Source: CAD feature listing. Evaluate the final solid. Frame: model axes, mm. Round coordinates to 2 decimals unless told otherwise and drop trailing zeros. Order: outer loops, then holes, each group sorted by start corner. A loop starts at its lowest first (then second) coordinate and runs counter-clockwise, first axis right, second up. Notation, with made-up numbers: M 17,74.5 L 56,74.5 A24 cw 56,84.5 Z; hole C 75,73.5 d2. An arc over 180 degrees is marked long. Use one line per item in the form item = value. Start each with the question number.
Q1. Section A-A (z = -131.5). Return the cut outline in (x, y).
Q2. Contact query for flat-ended pins moving along their axis: pin 1 (6 mm diameter, centred on x = 0, y = 0, fed in from +Z); pin 2 (6.5 mm diameter, centred on x = 0, z = 90, fed in from -Y). Output: stop coordinate, or through.
Q3. Material intervals for probe 1 along Y at (x, z) = (0, -138.5); probe 2 along X at (y, z) = (-1.25, 90); probe 3 along Z at (x, y) = (-0.5, -5), sorted ascending.
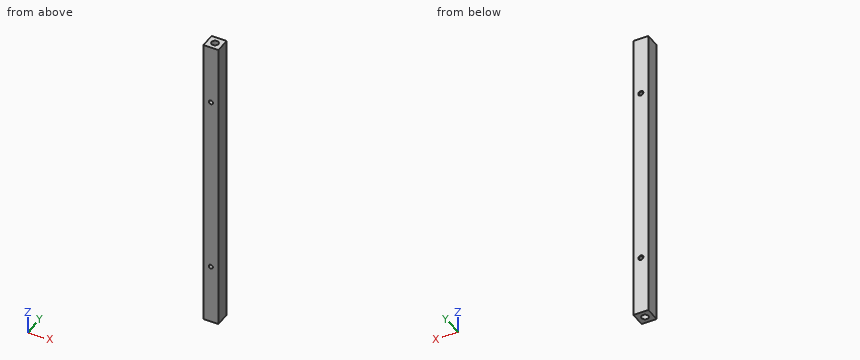
from build123d import *

# Parameters (mm, degrees)
IZIM1_W                     = 15
IZIM1_H                     = 15
Y_KSEKLIK_EKSTR_ZYON1_DEPTH = 150
M5_DI_LI_DELIK1_D           = 4.2
M5_DI_LI_DELIK1_CSINK_D     = 5.05
M5_DI_LI_DELIK1_CSINK_ANGLE = 90


with BuildPart() as part:
    # Çizim1 → Yükseklik-Ekstrüzyon1 (new, symmetric)
    with BuildSketch(Plane.XY):
        Rectangle(IZIM1_W, IZIM1_H)
    extrude(amount=Y_KSEKLIK_EKSTR_ZYON1_DEPTH, both=True)

    # Çizim3 → M8 Dişli Delik1 (revolve, cut)
    with BuildSketch(Plane(origin=(0, 0, 150), x_dir=(0, -1, 0), z_dir=(1, 0, 0))):
        Polygon((0, 0), (0, 24.292926105), (3.4, 22.25), (3.4, 0), align=None)
    m8_di_li_delik1 = revolve(axis=Axis((0, 0, 156.35), (0, 0, -1)), mode=Mode.SUBTRACT)

    # Aynalama1: M8 Dişli Delik1 across plane
    add(m8_di_li_delik1.mirror(Plane.XY), mode=Mode.SUBTRACT)

    # M5 Dişli Delik1 (through all)
    with Locations(Plane(origin=(0, 7.5, 0), x_dir=(1, 0, 0), z_dir=(0, 1, 0))):
        with Locations((0, 90)):
            m5_di_li_delik1 = CounterSinkHole(M5_DI_LI_DELIK1_D / 2, M5_DI_LI_DELIK1_CSINK_D / 2, counter_sink_angle=M5_DI_LI_DELIK1_CSINK_ANGLE)

    # Aynalama2: M5 Dişli Delik1 across plane
    add(m5_di_li_delik1.mirror(Plane.XY), mode=Mode.SUBTRACT)


solid = part.part
Results list:
q1.outline = M -7.5,-7.5 L 7.5,-7.5 L 7.5,7.5 L -7.5,7.5 Z; hole C 0,0 d6.8
q2.pin_1 = 127.51
q2.pin_2 = -7.5
q3.probe_1 = -7.5 to -3.4, 3.4 to 7.5
q3.probe_2 = -7.5 to -2.1, 2.1 to 7.5
q3.probe_3 = -150 to -92.04, -87.96 to 87.96, 92.04 to 150
